The listing builds one solid part. Answer for the finished solid, in the listing's coordinates (mm). A direction names the side the tool comes from. Coordinates: 2 decimals unless noted, no trailing zeros. Order: outer loops, then holes, each group sorted by start corner. A loop starts at its lowest first (then second) coordinate and runs counter-clockwise, first axis right, second up.
from build123d import *

# Parameters (mm, degrees)
SKETCH_R       = 18.7
PAD_DEPTH      = 24
SKETCH001_R    = 16
PAD001_DEPTH   = 30
SKETCH002_R    = 1
PAD002_DEPTH   = 12
SKETCH003_R    = 13
PAD003_DEPTH   = 16
SKETCH004_R    = 17.5
PAD004_DEPTH   = 11
SKETCH008_R    = 22
SKETCH008_R_2  = 12
PAD008_DEPTH   = 2.5
SKETCH007_R    = 22
SKETCH007_R_2  = 12
PAD007_DEPTH   = 2.5
SKETCH006_R    = 22
SKETCH006_R_2  = 16
PAD006_DEPTH   = 2.5
SKETCH005_R    = 22
SKETCH005_R_2  = 16
PAD005_DEPTH   = 2.5
CYLINDER_R     = 20
CYLINDER_DEPTH = 93
SKETCH012_R    = 17.5
SKETCH012_R_2  = 14.7
POCKET_DEPTH   = 1.5


with BuildPart() as obj1:
    # Sketch → Pad (new body)
    with BuildSketch(Plane.XY):
        Circle(SKETCH_R)
    extrude(amount=PAD_DEPTH)

    # Sketch001 → Pad001 (new body)
    with BuildSketch(Plane.XY.offset(24)):
        Circle(SKETCH001_R)
    extrude(amount=PAD001_DEPTH)

    # Sketch002 → Pad002 (new body)
    with BuildSketch(Plane.XY.offset(54)):
        with Locations((-9.2, 0)):
            Circle(SKETCH002_R)
    extrude(amount=PAD002_DEPTH)

    # Sketch003 → Pad003 (new body)
    with BuildSketch(Plane.XY.offset(66)):
        Circle(SKETCH003_R)
    extrude(amount=PAD003_DEPTH)

    # Sketch004 → Pad004 (new body)
    with BuildSketch(Plane.XY.offset(82)):
        Circle(SKETCH004_R)
    extrude(amount=PAD004_DEPTH)


with BuildPart() as pad008:
    # Sketch008 → Pad008 (new body)
    with BuildSketch(Plane.XY.offset(56)):
        Circle(SKETCH008_R)
        Circle(SKETCH008_R_2, mode=Mode.SUBTRACT)
    extrude(amount=PAD008_DEPTH)


with BuildPart() as pad007:
    # Sketch007 → Pad007 (new body)
    with BuildSketch(Plane.XY.offset(61)):
        Circle(SKETCH007_R)
        Circle(SKETCH007_R_2, mode=Mode.SUBTRACT)
    extrude(amount=PAD007_DEPTH)


with BuildPart() as pad006:
    # Sketch006 → Pad006 (new body)
    with BuildSketch(Plane.XY.offset(71)):
        Circle(SKETCH006_R)
        Circle(SKETCH006_R_2, mode=Mode.SUBTRACT)
    extrude(amount=PAD006_DEPTH)


with BuildPart() as pad005:
    # Sketch005 → Pad005 (new body)
    with BuildSketch(Plane.XY.offset(66)):
        Circle(SKETCH005_R)
        Circle(SKETCH005_R_2, mode=Mode.SUBTRACT)
    extrude(amount=PAD005_DEPTH)


with BuildPart() as nut_axial:
    # Cylinder → Cylinder (new body)
    with BuildSketch(Plane.XY):
        Circle(CYLINDER_R)
    extrude(amount=CYLINDER_DEPTH)

    # Cut: cut Pad005
    add(pad005.part, mode=Mode.SUBTRACT)

    # Cut001: cut Pad006
    add(pad006.part, mode=Mode.SUBTRACT)

    # Cut002: cut Pad007
    add(pad007.part, mode=Mode.SUBTRACT)

    # Cut003: cut Pad008
    add(pad008.part, mode=Mode.SUBTRACT)

    # Cut010: cut obj1
    add(obj1.part, mode=Mode.SUBTRACT)

    # Sketch012 → Pocket (cut)
    with BuildSketch(Plane.XY.offset(82)):
        Circle(SKETCH012_R)
        Circle(SKETCH012_R_2, mode=Mode.SUBTRACT)
    extrude(amount=-POCKET_DEPTH, mode=Mode.SUBTRACT)


solid = nut_axial.part
(1) Find section B-B on z = 17. Determine the outline of the cut face in (x, y), then the cut area to 3 significant figures.
(2) A tool of negligible diameter and unlimited length cuts with its end or side. For faces 5 (the cylindrical face through (-3.47, -15.62, 67.23)), 6 (the flat face through (0, -18, 93)), 7 (the cylindrical face through (-10.316, -7.91, 73.888)), 8 (the flat face through (0, 0, 54)), 9 (the cylindrical face through (-4.336, -19.524, 83.114)), from which of +Z, -Z, +X, -X, +Y, -Y can it reach the whole face along a straight path? Write none if from no direction.
(3) The mould has two halves that part along Y. Classify faces 1 (the cylindrical face through (-8.246, 0.3, 59.916)), 2 (the cylindrical face through (-4.336, -19.524, 64.732)), 3 (the cylindrical face through (-3.47, -15.62, 38.79)), 4 (the flat face through (9, -9, 61)): pulls with the +Y half, pulls with the -Y half, needs draft (parallel to the pull), parting line crosses it, or undercut.
(4) Find section A-A on z = 50. Determine the outline of the cut face in (x, y), then the cut area to 3 significant figures.
(5) Given pin 1 Ø23.5 at (x, y) = (0, 0) entering from +Z; pin 2 Ø1.5 at (y, z) = (2.5, 76.5) entering from -X; pin 3 Ø5 at (x, z) = (0, 64.5) entering from -Y, each flat-ended and moving along its own axis, determine where each tip first touches the part or whether it passes through.
(6) Find the intervals of material crossed by probe 1 along Z at (x, y) = (18, 1.5); probe 2 along Y at (x, z) = (0, 81.3); probe 3 along Z at (x, y) = (4, 12.5), in increasing order.
Resolved:
1. outline: circle Ø40 at (0, 0); hole circle Ø37.4 at (0, 0)
1. area: 158 mm2
2. face 5: none
2. face 6: +Z, +X, -X, +Y, -Y
2. face 7: +Z
2. face 8: -Z
2. face 9: +Z, -Z
3. face 1: undercut
3. face 2: parting line crosses it
3. face 3: undercut
3. face 4: needs draft
4. outline: circle Ø40 at (0, 0); hole circle Ø32 at (0, 0)
4. area: 452 mm2
5. pin 1: stops at z = 66
5. pin 2: stops at x = -19.92
5. pin 3: stops at y = -20
6. probe 1: z = 24 to 56, 58.5 to 61, 63.5 to 66, 68.5 to 71, 73.5 to 93
6. probe 2: y = -20 to -17.5, -14.7 to -13, 13 to 14.7, 17.5 to 20
6. probe 3: z = 54 to 56, 58.5 to 61, 63.5 to 82
